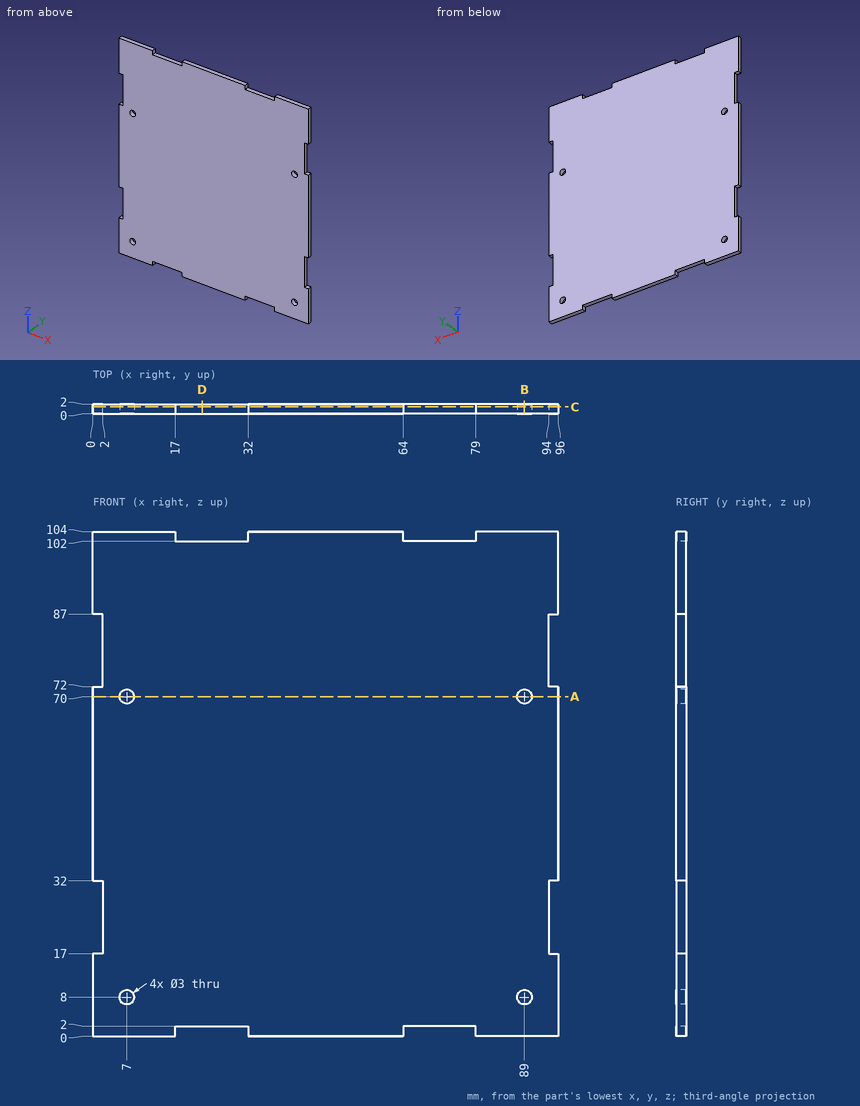
Here's the drawing with two shaded views (mm, measured from the low corner). I have some questions. Coordinates: 2 decimals unless noted, no trailing zeros. Order: outer loops, then holes, each group sorted by start corner. A loop starts at its lowest first (then second) coordinate and runs counter-clockwise, first axis right, second up. Notation, with made-up numbers: (20.25, 57.25) - (63.25, 57.25) arc R17 ccw to (63.25, 61.25) - close; hole circle Ø5 at (9, -13). An arc over 180 degrees is marked (long way). Answer in a Markdown table with one row per item. Add a question column.
(1) If we section it at B-B, the plane x = 89: Please give me the cut outline in (y, z), then the cut area to 3 significant figures.
(2) I need wall thicknesses on L1, parallel to Z at x = 7, y = 0.9; L2, parallel to X at y = 1.45, z = 70; L3, parallel to X at y = 1.9, z = 7.5. Which ranges of each line are inside material? Lowest first, please.
(3) If we section it at C-C, the plane y = 1.4: State how many separate pieces and enclosed holes the cut face has, then the cut area to 3 significant figures.
(4) Will these pins go through, and if not, where does the flat tip stop? pin 1 (1.8 mm diameter, centred on x = 89, z = 70, fed in from -Y); pin 2 (0.6 mm diameter, centred on y = 1.5, z = 82, fed in from +X); pin 3 (0.6 mm diameter, centred on x = 73, y = 1.5, fed in from +Z); pin 4 (1 mm diameter, centred on y = 0.5, z = 28, fed in from -X).
(5) If we section it at A-A, the plane z = 70: Please give me the cut outline in (x, y).
(6) If we section it at D-D, the plane x = 22.5: Please give me the cut outline in (y, z), then the cut area to 3 significant figures.
Results are:
| question | item | result |
|---|---|---|
| 1 | outline | (0, 0) - (2, 0) - (2, 6.5) - (0, 6.5) - close; (0, 9.5) - (2, 9.5) - (2, 68.5) - (0, 68.5) - close; (0, 71.5) - (2, 71.5) - (2, 104) - (0, 104) - close |
| 1 | area | 196 mm2 |
| 2 | L1 | z = 0 to 6.5, 9.5 to 68.5, 71.5 to 104 |
| 2 | L2 | x = 0 to 5.5, 8.5 to 87.5, 90.5 to 96 |
| 2 | L3 | x = 0 to 5.59, 8.41 to 87.59, 90.41 to 96 |
| 3 | separate pieces | 1 |
| 3 | enclosed holes | 4 |
| 3 | area | 9,720 mm2 |
| 4 | pin 1 | passes through |
| 4 | pin 2 | stops at x = 94 |
| 4 | pin 3 | stops at z = 102 |
| 4 | pin 4 | stops at x = 2 |
| 5 | outline | (0, 0) - (5.5, 0) - (5.5, 2) - (0, 2) - close; (8.5, 0) - (87.5, 0) - (87.5, 2) - (8.5, 2) - close; (90.5, 0) - (96, 0) - (96, 2) - (90.5, 2) - close |
| 6 | outline | (0, 2) - (2, 2) - (2, 102) - (0, 102) - close |
| 6 | area | 200 mm2 |
